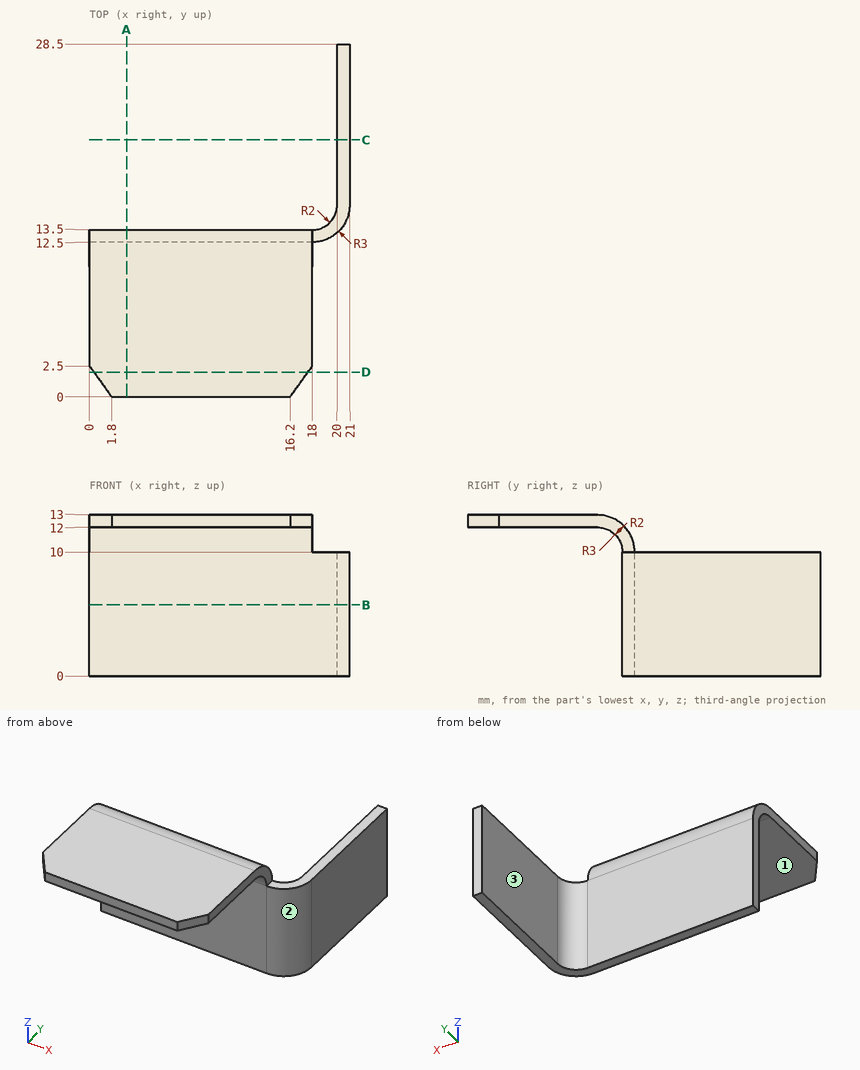
Could you check a few things on this drawing? It's one solid part, dimensions in mm from its lowest x, y, z. A direction names the side the tool comes from. Round coordinates to 2 decimals unless told otherwise and drop trailing zeros. Loops run counter-clockwise (first coordinate to the right, second up) from the corner with the lowest first, then second, coordinate; pieces in that order, holes last.
Q1. For P1, Ø1.5, axis at x = 20, y = 21, coming from the +Z side; P2, Ø1.5, axis at x = 4.5, z = 1.5, coming from the -Y side; P3, Ø5, axis at x = 5, y = 4, coming from the -Z side, each with a flat end and sliding along its axis, tell me the tip position at first contact or that it passes through.
Q2. I want a section at B-B (z = 5.75). Write out the boundary of the cut face in (x, y).
Q3. I want a section at D-D (y = 2). Write out the boundary of the cut face in (x, z).
Q4. Please list where these lines run through material, in increasing order: L1, parallel to X at y = 21.25, z = 3.25; L2, parallel to Y at x = 1, z = 3.75; L3, parallel to Z at x = 4.25, y = 2.25.
Q5. I want a section at A-A (x = 3). Write out the boundary of the cut face in (y, z), and give its area (3 significant figures).
Q6. On a 3-axis mill with a long thin cutter (end or side, diameter ignored), from which of +Z, -Z, +X, -X, +Y, -Y can I reach the whole of each face in a straight line? I mean the marked faces 1, 2 and 3. Say none if no direction works.
Q7. I want a section at C-C (y = 20.75). Write out the boundary of the cut face in (x, z), and give its area (3 significant figures).
Answer below:
1. P1: stops at z = 10
1. P2: stops at y = 12.5
1. P3: stops at z = 12
2. outline: (0, 12.5) - (18, 12.5) arc R3 ccw to (21, 15.5) - (21, 28.5) - (20, 28.5) - (20, 15.5) arc R2 cw to (18, 13.5) - (0, 13.5) - close
3. outline: (0.36, 12) - (17.64, 12) - (17.64, 13) - (0.36, 13) - close
4. L1: x = 20 to 21
4. L2: y = 12.5 to 13.5
4. L3: z = 12 to 13
5. outline: (0, 12) - (10.5, 12) arc R2 cw to (12.5, 10) - (12.5, 0) - (13.5, 0) - (13.5, 10) arc R3 ccw to (10.5, 13) - (0, 13) - close
5. area: 24.4 mm2
6. face 1: -Z, +X, -X, -Y
6. face 2: +Z, -Z, +X, -Y
6. face 3: +Z, -Z, -X, +Y
7. outline: (20, 0) - (21, 0) - (21, 10) - (20, 10) - close
7. area: 10.0 mm2
